```python
from build123d import *

# Parameters (mm, degrees)
SKETCH1_R                           = 11.1125
BOSS_EXTRUDE1_DEPTH                 = 12.7
CUT_EXTRUDE1_START                  = -12.7
SKETCH2_R                           = 4.25
CUT_EXTRUDE1_DEPTH                  = 12.7
CUT_EXTRUDE2_START                  = -12.7
SKETCH3_R                           = 4.8895
CUT_EXTRUDE2_DEPTH                  = 12.7
CUT_EXTRUDE3_REACH                  = 31.869
CUT_EXTRUDE4_DEPTH                  = 4
CUT_EXTRUDE4_DIRECTION_2_REACH      = 26.756
CUT_EXTRUDE4_DIRECTION_2_END_RADIUS = 11.1125
M3_CLEARANCE_HOLE1_D                = 3.4
CUT_EXTRUDE5_REACH                  = 23.999
SKETCH9_R                           = 3.5


with BuildPart() as part:
    # Sketch1 → Boss-Extrude1 (new, symmetric)
    with BuildSketch(Plane(origin=(0, 0, 0), x_dir=(1, 0, 0), z_dir=(0, 1, 0))):
        with Locations(Location((0, 0, 0), (0, 0, 270))):
            Circle(SKETCH1_R)
    extrude(amount=BOSS_EXTRUDE1_DEPTH, both=True)

    # Sketch2 → Cut-Extrude1 (cut)
    with BuildSketch(Plane(origin=(0, 12.7, 0), x_dir=(1, 0, 0), z_dir=(0, 1, 0)).offset(CUT_EXTRUDE1_START)):
        with Locations(Location((0, 0, 0), (0, 0, 270))):
            Circle(SKETCH2_R)
    extrude(amount=CUT_EXTRUDE1_DEPTH, mode=Mode.SUBTRACT)

    # Sketch3 → Cut-Extrude2 (cut)
    with BuildSketch(Plane.XZ.offset(12.7).offset(CUT_EXTRUDE2_START)):
        with Locations(Location((0, 0, 0), (0, 0, 270))):
            Circle(SKETCH3_R)
    extrude(amount=CUT_EXTRUDE2_DEPTH, mode=Mode.SUBTRACT)

    # Sketch4 → Cut-Extrude3 (cut, up to next)
    with BuildSketch(Plane(origin=(0, 12.7, 0), x_dir=(1, 0, 0), z_dir=(0, 1, 0)), mode=Mode.PRIVATE) as cut_extrude3_sk1:
        with BuildLine():
            Line((-1, 4.13067791), (-1, 11.067414163))
            ThreePointArc((-1, 11.067414163), (0, 11.1125), (1, 11.067414163))
            Line((1, 11.067414163), (1, 4.13067791))
            ThreePointArc((1, 4.13067791), (0, 4.25), (-1, 4.13067791))
        make_face()
    cut_extrude3_tool1 = extrude(cut_extrude3_sk1.sketch, amount=-CUT_EXTRUDE3_REACH, mode=Mode.PRIVATE) & part.part
    add(cut_extrude3_tool1.solids().sort_by_distance((0, 12.7, -7.653889))[0], mode=Mode.SUBTRACT)

    # Sketch5 → Cut-Extrude4 (cut)
    with BuildSketch(Plane(origin=(7, 0, 0), x_dir=(0, 0, -1), z_dir=(1, 0, 0))):
        Polygon((7.926780955, 2.885898385), (10.926780955, 4.617949192), (10.926780955, 8.082050808), (7.926780955, 9.814101615), (4.926780955, 8.082050808), (4.926780955, 4.617949192), align=None)
        Polygon((7.926780955, -9.814101615), (10.926780955, -8.082050808), (10.926780955, -4.617949192), (7.926780955, -2.885898385), (4.926780955, -4.617949192), (4.926780955, -8.082050808), align=None)
    extrude(amount=-CUT_EXTRUDE4_DEPTH, mode=Mode.SUBTRACT)

    # Cut-Extrude4 direction 2: up to this cylinder (the profile starts inside it)
    cut_extrude4_direction_2_end = Plane(origin=(0, 0, 0), z_dir=(0, -1, 0)) * Cylinder(CUT_EXTRUDE4_DIRECTION_2_END_RADIUS, 89.437, mode=Mode.PRIVATE)
    # Sketch5 → Cut-Extrude4 direction 2 (cut, up to the surface)
    with BuildSketch(Plane(origin=(7, 0, 0), x_dir=(0, 0, -1), z_dir=(1, 0, 0)), mode=Mode.PRIVATE) as cut_extrude4_direction_2_sk1:
        Polygon((7.926780955, 2.885898385), (10.926780955, 4.617949192), (10.926780955, 8.082050808), (7.926780955, 9.814101615), (4.926780955, 8.082050808), (4.926780955, 4.617949192), align=None)
    cut_extrude4_direction_2_tool1 = extrude(cut_extrude4_direction_2_sk1.sketch, amount=CUT_EXTRUDE4_DIRECTION_2_REACH, mode=Mode.PRIVATE) & cut_extrude4_direction_2_end
    add(cut_extrude4_direction_2_tool1.solids().sort_by_distance((7, 6.35, -7.926781))[0], mode=Mode.SUBTRACT)
    # Sketch5 → Cut-Extrude4 direction 2 (cut, up to the surface)
    with BuildSketch(Plane(origin=(7, 0, 0), x_dir=(0, 0, -1), z_dir=(1, 0, 0)), mode=Mode.PRIVATE) as cut_extrude4_direction_2_sk2:
        Polygon((7.926780955, -9.814101615), (10.926780955, -8.082050808), (10.926780955, -4.617949192), (7.926780955, -2.885898385), (4.926780955, -4.617949192), (4.926780955, -8.082050808), align=None)
    cut_extrude4_direction_2_tool2 = extrude(cut_extrude4_direction_2_sk2.sketch, amount=CUT_EXTRUDE4_DIRECTION_2_REACH, mode=Mode.PRIVATE) & cut_extrude4_direction_2_end
    add(cut_extrude4_direction_2_tool2.solids().sort_by_distance((7, -6.35, -7.926781))[0], mode=Mode.SUBTRACT)

    # M3 Clearance Hole1 (through all)
    with Locations(Plane(origin=(3, 0, 0), x_dir=(0, 0, -1), z_dir=(1, 0, 0))):
        with Locations((7.926780955, 6.35), (7.926780955, -6.35)):
            Hole(M3_CLEARANCE_HOLE1_D / 2)

    # Sketch9 → Cut-Extrude5 (cut, up to next)
    with BuildSketch(Plane(origin=(-3, 0, 0), x_dir=(0, 0, -1), z_dir=(1, 0, 0)), mode=Mode.PRIVATE) as cut_extrude5_sk1:
        with Locations((7.926780955, 6.35)):
            Circle(SKETCH9_R)
    cut_extrude5_tool1 = extrude(cut_extrude5_sk1.sketch, amount=-CUT_EXTRUDE5_REACH, mode=Mode.PRIVATE) & part.part
    # Sketch9 → Cut-Extrude5 (cut, up to next)
    with BuildSketch(Plane(origin=(-3, 0, 0), x_dir=(0, 0, -1), z_dir=(1, 0, 0)), mode=Mode.PRIVATE) as cut_extrude5_sk2:
        with Locations((7.926780955, -6.35)):
            Circle(SKETCH9_R)
    cut_extrude5_tool2 = extrude(cut_extrude5_sk2.sketch, amount=-CUT_EXTRUDE5_REACH, mode=Mode.PRIVATE) & part.part
    add(cut_extrude5_tool1.solids().sort_by_distance((-3, 6.35, -7.926781))[0], mode=Mode.SUBTRACT)
    add(cut_extrude5_tool2.solids().sort_by_distance((-3, -6.35, -7.926781))[0], mode=Mode.SUBTRACT)


solid = part.part
```
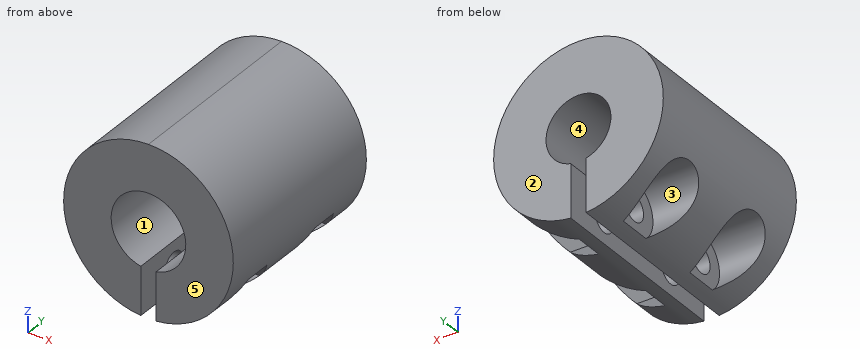
Could you check a few things on this model? Use its own coordinates, in mm. Face numbers are marked on the shaded views. A direction names the side the tool comes from. Give positions to 0.01 mm unless a question says otherwise; leave off trailing zeros. Loops run counter-clockwise (first coordinate to the right, second up) from the corner with the lowest first, then second, coordinate; pieces in that order, holes last. Notation, with made-up numbers: (44.5, 30) -> (54.5, 30) arc R23 ccw to (54.5, 62) -> close; hole circle Ø8 at (-17, -11). An arc over 180 degrees is marked (long way). Put each result on its own line as item: value.
(1) Imagine slicing it at D-D on y = 6.35. State how many separate pieces and enclosed holes the cut face has, plus the area to 3 significant figures.
Computed:
separate pieces: 3
enclosed holes: 0
area: 248 mm^2
(2) Please list where these lines run through material, in increasing order: probe 1 along X at (y, z) = (5, 0); probe 2 along X at (y, z) = (-8, 0); probe 3 along Z at (x, y) = (2.75, 5). Write a range as [from, to].
Computed:
probe 1: [-11.11, -4.25], [4.25, 11.11]
probe 2: [-11.11, -4.89], [4.89, 11.11]
probe 3: [-10.77, -8.96], [-6.89, -3.24], [3.24, 10.77]
(3) Imagine slicing it at A-A on y = -6.35. Write out the boundary of the cut face in (x, z) (1 decimal).
Computed:
outline: (-10.2, -4.4) -> (-3, -4.4) -> (-3, -6.2) -> (-1, -6.2) -> (-1, -4.8) arc R4.9 cw (long way) to (1, -4.8) -> (1, -6.2) -> (3, -6.2) -> (3, -4.9) -> (10, -4.9) arc R11.1 ccw (long way) to start; (-3, -10.7) arc R11.1 ccw to (-1, -11.1) -> (-1, -9.6) -> (-3, -9.6) -> close; (1, -11.1) arc R11.1 ccw to (3, -10.7) -> (3, -9.6) -> (1, -9.6) -> close
(4) For the marked faces 1, 2 and 3, which set-ups out of +Z, -Z, +X, -X, +Y, -Y let a thin tool reach every point of the face, with its end or its side?
Computed:
face 1: -Y
face 2: +Z, -Z, +X, -X, +Y
face 3: -X
(5) Imagine slicing it at B-B on x = -2. Write out the boundary of the cut face in (y, z).
Computed:
outline: (-12.7, -10.93) -> (12.7, -10.93) -> (12.7, -3.75) -> (0, -3.75) -> (0, -4.46) -> (-12.7, -4.46) -> close; (-12.7, 4.46) -> (0, 4.46) -> (0, 3.75) -> (12.7, 3.75) -> (12.7, 10.93) -> (-12.7, 10.93) -> close; hole circle Ø3.4 at (-6.35, -7.93); hole circle Ø3.4 at (6.35, -7.93)
(6) Imagine slicing it at C-C on z = 0. Write out the boundary of the cut face in (x, y).
Computed:
outline: (-11.11, -12.7) -> (-4.89, -12.7) -> (-4.89, 0) -> (-4.25, 0) -> (-4.25, 12.7) -> (-11.11, 12.7) -> close; (4.25, 0) -> (4.89, 0) -> (4.89, -12.7) -> (11.11, -12.7) -> (11.11, 12.7) -> (4.25, 12.7) -> close
(7) I'm going to push flat-ended pins straight in: pin 1 Ø11 at (y, z) = (-6.35, -7.93) entering from -X; pin 2 Ø3.5 at (y, z) = (-5.5, -6.5) entering from -X; pin 3 Ø3 at (y, z) = (-4.5, 0.5) entering from +X; pin 4 Ø8 at (y, z) = (-9.5, -6) entering from -X. Where does each tip first touch, or does it pass through?
Computed:
pin 1: x = -10.84
pin 2: x = -3
pin 3: x = 11.11
pin 4: x = -10.93
(8) Thinking about a two-plate mould opening in Z: for the marked faces 4 and 5, which applies, pulls with the +Z half, pulls with the -Z half, needs draft (parallel to the pull), parting line crosses it, or undercut?
Computed:
face 4: undercut
face 5: needs draft
